Geometry check sheet. Reference: drawing and pictorial views, mm from the part's lowest x, y, z. A direction names the side the tool comes from. Give positions to 0.01 mm unless a question says otherwise; leave off trailing zeros.
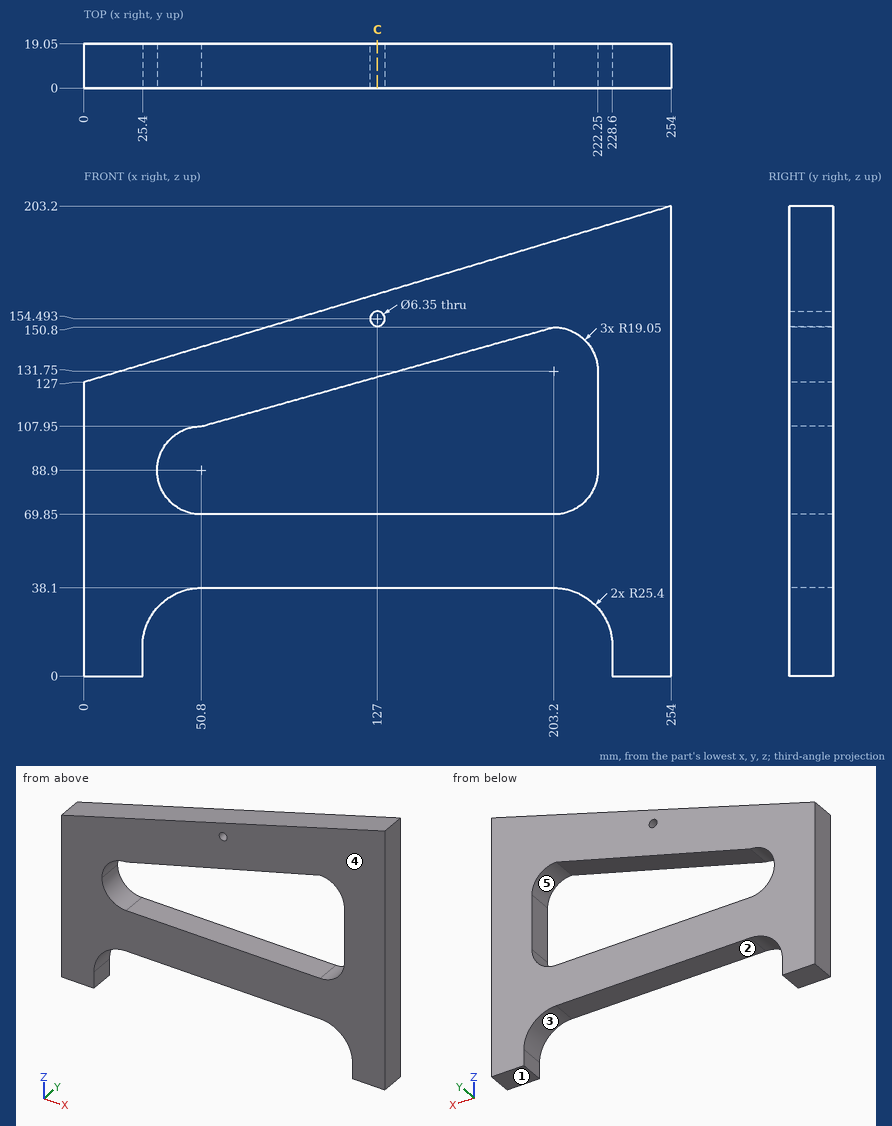
(1) Material ranges on L1, parallel to Z at x = 46.5, y = 17.5; L2, parallel to X at y = 2, z = 83; L3, parallel to X at y = 8.5, z = 35, recorded low to high.
Response values:
L1: z = 37.73 to 70.34, 107.46 to 140.95
L2: x = 0 to 32.69, 221.31 to 254
L3: x = 0 to 38.64, 215.36 to 254
(2) Gauge pin test, flat ends, axial feed: pin 1 Ø1 at (x, y) = (103.5, 13) entering from +Z; pin 2 Ø5.5 at (x, z) = (127, 154.49) entering from -Y; pin 3 Ø4 at (x, y) = (168.5, 8) entering from +Z; pin 4 Ø6 at (x, y) = (54.5, 17) entering from -Z. Record the tip position at first contact, or that the pin passes through.
Response values:
pin 1: stops at z = 158.2
pin 2: passes through
pin 3: stops at z = 178.15
pin 4: stops at z = 38.1
(3) Release check for a two-part mould opening along X. For the marked faces 1 and 2 record: released by +X, released by -X, zero draft, split by the parting line, or undercut.
Response values:
face 1: zero draft
face 2: undercut
(4) Cross-section at C-C on x = 127. Count the separate pieces of the cut face and the enclosed holes in it, then the cut area to 3 significant figures.
Response values:
separate pieces: 3
enclosed holes: 0
area: 1,160 mm2
(5) Set-up check for the marked faces 3, 4 and 5: record each of +Z, -Z, +X, -X, +Y, -Y from which the full face is reachable in a straight line by a thin tool's end or side.
Response values:
face 3: -Z, +Y, -Y
face 4: +Z, -Z, +X, -X, -Y
face 5: +Y, -Y
